Verification items for this drawing (mm, ordinates from the low corner). A direction names the side the tool comes from. Coordinates: 2 decimals unless noted, no trailing zeros. Order: outer loops, then holes, each group sorted by start corner. A loop starts at its lowest first (then second) coordinate and runs counter-clockwise, first axis right, second up. Notation, with made-up numbers: M 15.5,67 L 25.5,67 A11 cw 25.5,84 Z; hole C 29.5,63 d9. An arc over 180 degrees is marked long. Answer as a JSON object with one key per item and string values. Group by question number.
(1) Cross-section at B-B (x = 1.25). Enter the section's corners in (y, z).
(2) Cross-section at A-A (y = 1.9). Enter the section's corners in (x, z), plus the area to 3 significant figures.
(3) Access from +Z, -Z, +X, -X, +Y, -Y to the whole of each face (thin tool, end or side, straight path). Record for the marked faces 1 and 2.
(4) Gauge pin test, flat ends, axial feed: pin 1 Ø1 at (x, z) = (2.5, 1.5) entering from -Y; pin 2 Ø1 at (y, z) = (1, 2.5) entering from +X; pin 3 Ø0.8 at (x, y) = (1.5, 1.5) entering from +Z. Record the tip position at first contact, or that the pin passes through.
(5) Cross-section at C-C (z = 2.75). Enter the section's corners in (x, y), plus the area to 3 significant figures.
(6) Mould release check, pull along Z, two halves, no side actions. Record for the marked faces 3, 4 and 5: released by +Z, released by -Z, zero draft, split by the parting line, or undercut.
(7) Material ranges on line 1 (X direction, y = 1.6, z = 2.25); line 2 (Z direction, x = 1.25, y = 2.4), recorded low to high.
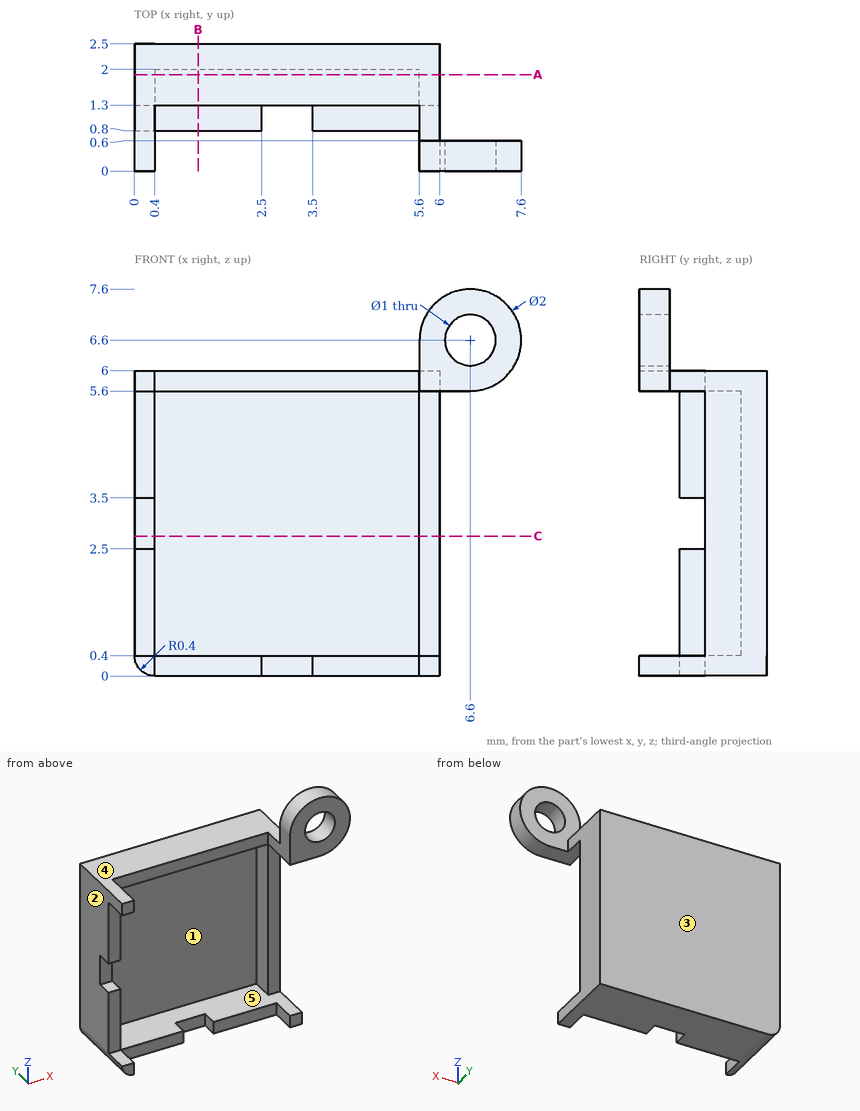
Taken from the geometry:
{
 "1": {"outline": "M 0.8,0 L 2.5,0 L 2.5,6 L 1.3,6 L 1.3,5.6 L 2,5.6 L 2,0.4 L 0.8,0.4 Z"},
 "2": {"outline": "M 0,0.4 A0.4 ccw 0.4,0 L 6,0 L 6,6 L 0,6 Z; hole M 0.4,0.4 L 5.6,0.4 L 5.6,5.6 L 0.4,5.6 Z", "area": "8.93 mm²"},
 "3": {"face 1": "-Y", "face 2": "+Z, -Z, -X, +Y, -Y"},
 "4": {"pin 1": "stops at y = 2", "pin 2": "stops at x = 6", "pin 3": "stops at z = 6"},
 "5": {"outline": "M 0,1.3 L 0.4,1.3 L 0.4,2 L 5.6,2 L 5.6,1.3 L 6,1.3 L 6,2.5 L 0,2.5 Z", "area": "3.56 mm²"},
 "6": {"face 3": "zero draft", "face 4": "released by +Z", "face 5": "undercut"},
 "7": {"line 1": "x = 0 to 0.4, 5.6 to 6", "line 2": "z = 0 to 6"}
}
